```python
from build123d import *

# Parameters (mm, degrees)
SKETCH1_R               = 41.9
SKETCH1_R_2             = 36.9
BOSS_EXTRUDE1_DEPTH     = 810
CUT_EXTRUDE_THIN1_START = -130
CUT_EXTRUDE_THIN1_DEPTH = 130
SKETCH3_R               = 36.9
BOSS_EXTRUDE2_DEPTH     = 2


# Read off the part's stored shape, not the designer's step: Cut-Extrude-Thin1
with BuildPart() as part:
    # Sketch1 → Boss-Extrude1 (new body)
    with BuildSketch(Plane(origin=(0, 0, 0), x_dir=(0, 0, -1), z_dir=(1, 0, 0))):
        Circle(SKETCH1_R)
        Circle(SKETCH1_R_2, mode=Mode.SUBTRACT)
    extrude(amount=BOSS_EXTRUDE1_DEPTH)

    # Cut-Extrude-Thin1 outline → Cut-Extrude-Thin1 (cut)
    with BuildSketch(Plane.ZY.offset(CUT_EXTRUDE_THIN1_START)):
        with BuildLine():
            ThreePointArc((-31.179923269, -19.733787901), (-31.9563374, -18.45), (-32.67992327, -17.135711689))
            Line((-32.67992327, -17.135711689), (-37.013204492, -19.637532769))
            ThreePointArc((-37.013204492, -19.637532769), (-36.286464419, -20.95), (-35.513204492, -22.235608981))
            Line((-35.513204492, -22.235608981), (-31.179923269, -19.733787901))
        make_face()
        with BuildLine():
            Line((-1.5, 41.87314175), (-1.5, 36.86949959))
            ThreePointArc((-1.5, 36.86949959), (0, 36.9), (1.5, 36.86949959))
            Line((1.5, 36.86949959), (1.5, 41.87314175))
            ThreePointArc((1.5, 41.87314175), (0, 41.9), (-1.5, 41.87314175))
        make_face()
        with BuildLine():
            ThreePointArc((32.67992327, -17.135711689), (31.9563374, -18.45), (31.179923269, -19.733787901))
            Line((31.179923269, -19.733787901), (35.513204492, -22.235608981))
            ThreePointArc((35.513204492, -22.235608981), (36.286464419, -20.95), (37.013204492, -19.637532769))
            Line((37.013204492, -19.637532769), (32.67992327, -17.135711689))
        make_face()
    extrude(amount=CUT_EXTRUDE_THIN1_DEPTH, mode=Mode.SUBTRACT)

    # Sketch3 → Boss-Extrude2 (add)
    with BuildSketch(Plane(origin=(610, 0, 0), x_dir=(0, 0, -1), z_dir=(1, 0, 0))):
        with Locations(Location((0, 0, 0), (0, 0, 207.67026134))):
            Circle(SKETCH3_R)
    extrude(amount=BOSS_EXTRUDE2_DEPTH)


solid = part.part
```
Build history of the part. All positions in model axes, mm. A direction names the side the tool comes from. Give positions to 0.01 mm unless a question says otherwise; leave off trailing zeros. Loops run counter-clockwise (first coordinate to the right, second up) from the corner with the lowest first, then second, coordinate; pieces in that order, holes last. Notation, with made-up numbers: (71, -29.5) - (87, -29.5) arc R17 ccw to (87, -21.5) - close; hole circle Ø6 at (-32, -38.5). An arc over 180 degrees is marked (long way). Use a Markdown table: item, result.
(1) Wall check: line 1 along Z through (x, y) = (277.5, 0); line 2 along X through (y, z) = (-10.5, 19.5). Give the ranges that are in metal, low to high.
Taken from the geometry:
| item | result |
|---|---|
| line 1 | -41.9 to -36.9, 36.9 to 41.9 |
| line 2 | 610 to 612 |
(2) Drop flat-ended pins along their axis: pin 1 Ø4 at (y, z) = (-10.5, 27.5) entering from -X; pin 2 Ø5 at (x, z) = (696, -1) entering from -Y; pin 3 Ø5.5 at (x, y) = (90, 38.5) entering from -Z. Give the stop position or say it passes through.
Taken from the geometry:
| item | result |
|---|---|
| pin 1 | x = 610 |
| pin 2 | y = -41.9 |
| pin 3 | z = -21.85 |
(3) Band-saw the part on A-A (x = 103). Give the cut face in (y, z), and give its area (3 significant figures).
Taken from the geometry:
| item | result |
|---|---|
| outline | (-22.24, -35.51) - (-19.73, -31.18) arc R36.9 cw to (-19.73, 31.18) - (-22.24, 35.51) arc R41.9 ccw to start; (-19.64, -37.01) arc R41.9 ccw to (41.87, -1.5) - (36.87, -1.5) arc R36.9 cw to (-17.14, -32.68) - close; (-19.64, 37.01) - (-17.14, 32.68) arc R36.9 cw to (36.87, 1.5) - (41.87, 1.5) arc R41.9 ccw to start |
| area | 1,190 mm2 |
(4) Band-saw the part on C-C (z = -13). Give the cut face in (x, y).
Taken from the geometry:
| item | result |
|---|---|
| outline | (0, -39.83) - (810, -39.83) - (810, -34.53) - (612, -34.53) - (612, 34.53) - (810, 34.53) - (810, 39.83) - (0, 39.83) - (0, 34.53) - (610, 34.53) - (610, -34.53) - (0, -34.53) - close |
(5) Which spindle directions (+Z, -Z, +X, -X, +Y, -Y) get a long thin tool onto all of the face, cutting with end or side? Do faces 4 (the face through (0, 20, -32)), 5 (the face through (612, 0, -1)), 6 (the face through (610, 0, -1)). Say none if no direction does.
Taken from the geometry:
| item | result |
|---|---|
| face 4 | +Z, -Z, -X, +Y, -Y |
| face 5 | +X |
| face 6 | -X |
(6) Pull direction Y, two halves, no side cores. Call faces 1 (the face through (300.73, 11.084, -35.196)), 2 (the face through (399.33, -37.173, -19.334)), 3 (the face through (0, -37.3, 0.2)): +Y half, -Y half, draft (parallel to the pull), parting line (faces both ways), or undercut.
Taken from the geometry:
| item | result |
|---|---|
| face 1 | undercut |
| face 2 | parting line |
| face 3 | draft |
(7) Band-saw the part on B-B (y = 0). Give the cut face in (x, z), and give its area (3 significant figures).
Taken from the geometry:
| item | result |
|---|---|
| outline | (0, -41.9) - (810, -41.9) - (810, -36.9) - (612, -36.9) - (612, 36.9) - (810, 36.9) - (810, 41.9) - (0, 41.9) - (0, 36.9) - (610, 36.9) - (610, -36.9) - (0, -36.9) - close |
| area | 8,250 mm2 |
(8) Band-saw the part on D-D (x = 390). Give the cut face in (y, z), and give its area (3 significant figures).
Taken from the geometry:
| item | result |
|---|---|
| outline | circle Ø83.8 at (0, 0); hole circle Ø73.8 at (0, 0) |
| area | 1,240 mm2 |
